Verification items for the finished model (mm, model axes). Coordinates: 2 decimals unless noted, no trailing zeros. Order: outer loops, then holes, each group sorted by start corner. A loop starts at its lowest first (then second) coordinate and runs counter-clockwise, first axis right, second up. Notation, with made-up numbers: M -27,25 L -3,25 A12 cw -3,32 Z; hole C 84,63.5 d9. An arc over 180 degrees is marked long. Return JSON: item names as keys, results as strings. Group by question number.
1. Gauge pin test, flat ends, axial feed: pin 1 (3 mm diameter, centred on x = -2, z = 36.5, fed in from -Y); pin 2 (2 mm diameter, centred on y = 2.5, z = 21, fed in from -X); pin 3 (1.5 mm diameter, centred on y = -1, z = 26.5, fed in from -X); pin 4 (3.5 mm diameter, centred on x = 6.35, y = 0, fed in from -Z). Record the tip position at first contact, or that the pin passes through.
2. Material ranges on line 1 along Z through (x, y) = (-1.75, 4.5); line 2 along Y through (x, z) = (-6.35, 65.25); line 3 along X through (y, z) = (-0.25, 28), recorded low to high.
3. Section check C-C, the plane z = 9. Record the cut outline in (x, y).
4. Section check A-A, the plane x = 0. Record the cut outline in (y, z), plus the area to 3 significant figures.
5. Section check D-D, the plane x = -6.35. Record the cut outline in (y, z), plus the area to 3 significant figures.
6. Section check B-B, the plane y = 0. Record the cut outline in (x, z).
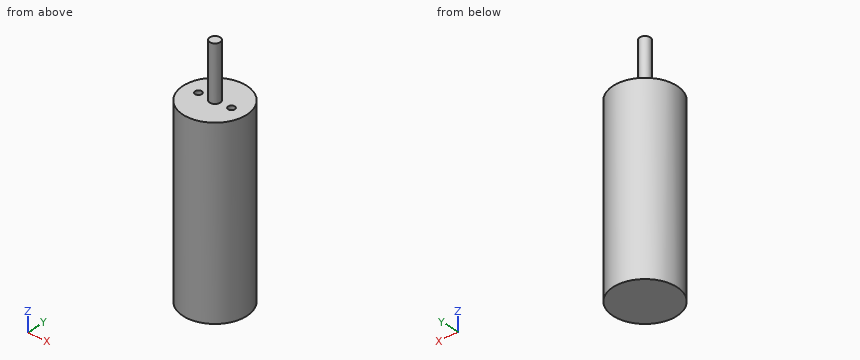
```python
from build123d import *

# Parameters (mm, degrees)
SKETCH1_R           = 12.192
BOSS_EXTRUDE1_DEPTH = 69.85
SKETCH2_R           = 2.032
BOSS_EXTRUDE2_DEPTH = 21
SKETCH3_R           = 1.27
CUT_EXTRUDE1_DEPTH  = 11.43


with BuildPart() as part:
    # Sketch1 → Boss-Extrude1 (new body)
    with BuildSketch(Plane.XY):
        Circle(SKETCH1_R)
    extrude(amount=BOSS_EXTRUDE1_DEPTH)

    # Sketch2 → Boss-Extrude2 (add)
    with BuildSketch(Plane.XY.offset(69.85)):
        with Locations(Location((0, 0, 0), (0, 0, 180))):
            Circle(SKETCH2_R)
    extrude(amount=BOSS_EXTRUDE2_DEPTH)

    # Sketch3 → Cut-Extrude1 (cut)
    with BuildSketch(Plane.XY.offset(69.85)):
        with Locations((6.35, 0)):
            Circle(SKETCH3_R)
        with Locations((-6.35, 0)):
            Circle(SKETCH3_R)
    extrude(amount=-CUT_EXTRUDE1_DEPTH, mode=Mode.SUBTRACT)


solid = part.part
```
Answers follow:
{
 "1": {"pin 1": "y = -12.18", "pin 2": "x = -12.1", "pin 3": "x = -12.19", "pin 4": "z = 0"},
 "2": {"line 1": "0 to 69.85", "line 2": "-10.41 to -1.27, 1.27 to 10.41", "line 3": "-12.19 to 12.19"},
 "3": {"outline": "C 0,0 d24.38"},
 "4": {"outline": "M -12.19,0 L 12.19,0 L 12.19,69.85 L 2.03,69.85 L 2.03,90.85 L -2.03,90.85 L -2.03,69.85 L -12.19,69.85 Z", "area": "1,790 mm^2"},
 "5": {"outline": "M -10.41,0 L 10.41,0 L 10.41,69.85 L 1.27,69.85 L 1.27,58.42 L -1.27,58.42 L -1.27,69.85 L -10.41,69.85 Z", "area": "1,420 mm^2"},
 "6": {"outline": "M -12.19,0 L 12.19,0 L 12.19,69.85 L 7.62,69.85 L 7.62,58.42 L 5.08,58.42 L 5.08,69.85 L 2.03,69.85 L 2.03,90.85 L -2.03,90.85 L -2.03,69.85 L -5.08,69.85 L -5.08,58.42 L -7.62,58.42 L -7.62,69.85 L -12.19,69.85 Z"}
}
